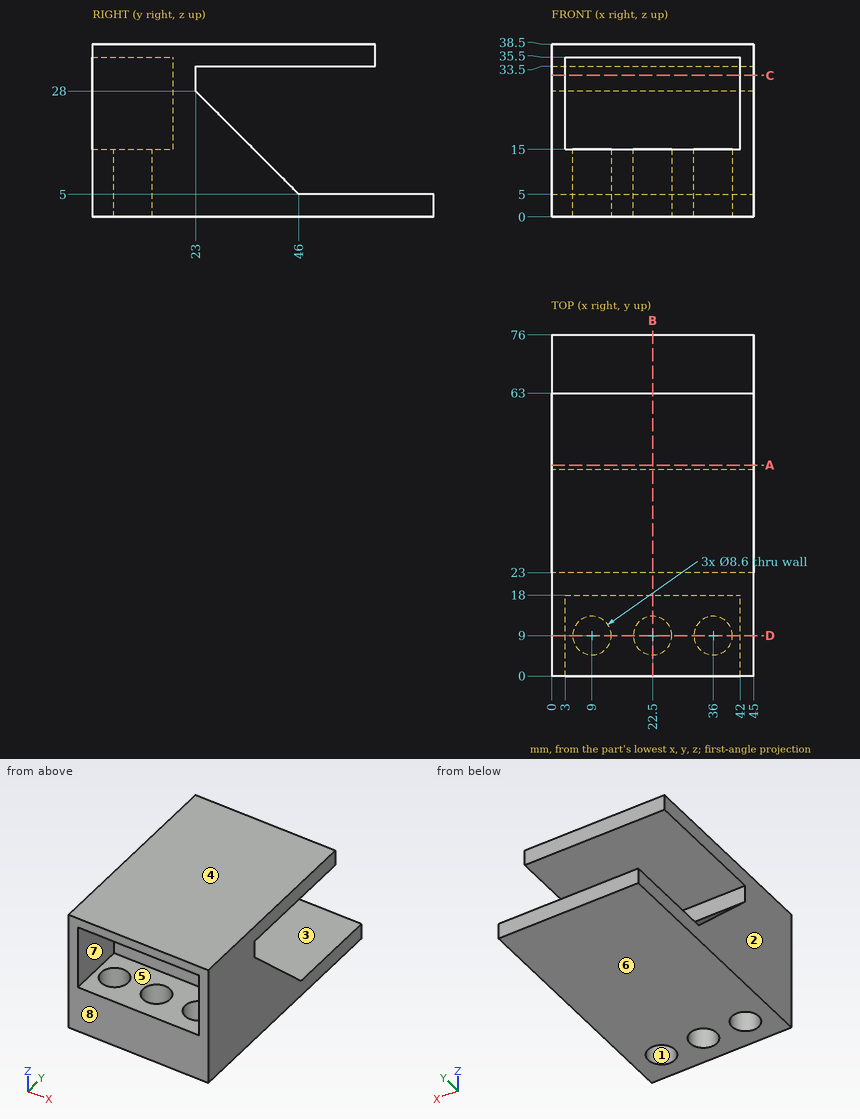
Job drawing, mm, ordinate dimensions from the low corner. One solid piece. A direction names the side the tool comes from. Give positions to 0.01 mm unless a question says otherwise; leave off trailing zeros. Order: outer loops, then holes, each group sorted by start corner. A loop starts at its lowest first (then second) coordinate and runs counter-clockwise, first axis right, second up. Notation, with made-up numbers: M -10,-0.5 L 5,-0.5 A25 cw 5,35.5 Z; hole C 17,-4 d8. An arc over 180 degrees is marked long. Return JSON: item names as keys, results as strings.
Q1. Wall check: probe 1 along Y at (x, z) = (22.5, 6); probe 2 along Z at (x, y) = (12, 61.5); probe 3 along Z at (x, y) = (38, 5). Give the ranges that are in metal, low to high. Write a range as from..to.
Answer list:
{"probe 1": "y = 0..4.7, 13.3..45", "probe 2": "z = 0..5, 33.5..38.5", "probe 3": "z = 0..15, 35.5..38.5"}
Q2. Band-saw the part on D-D (y = 9). Give the cut face in (x, z), then the cut area to 3 significant figures.
Answer list:
{"outline": "M 0,0 L 4.7,0 L 4.7,15 L 3,15 L 3,35.5 L 42,35.5 L 42,15 L 40.3,15 L 40.3,0 L 45,0 L 45,38.5 L 0,38.5 Z; M 13.3,0 L 18.2,0 L 18.2,15 L 13.3,15 Z; M 26.8,0 L 31.7,0 L 31.7,15 L 26.8,15 Z", "area": "546 mm^2"}
Q3. Band-saw the part on C-C (z = 31.5). Give the cut face in (x, y).
Answer list:
{"outline": "M 0,0 L 3,0 L 3,18 L 42,18 L 42,0 L 45,0 L 45,23 L 0,23 Z"}
Q4. Flat gauge pins, fed straight in: pin 1 (20 mm diameter, centred on x = 17, y = 13.5, fed in from -Z); pin 2 (1.5 mm diameter, centred on x = 22, z = 37, fed in from +Y); pin 3 (10 mm diameter, centred on x = 29, z = 22.5, fed in from -Y); pin 4 (8 mm diameter, centred on x = 28, z = 20, fed in from +Y). Where does each tip first touch, or does it go through?
Answer list:
{"pin 1": "stops at z = 0", "pin 2": "stops at y = 63", "pin 3": "stops at y = 18", "pin 4": "stops at y = 35"}
Q5. 3-axis set-ups, long thin cutter, end or side, ignore diameter. For the marked faces 1, 2, 3, 4 and 5: which of +Z, -Z, +X, -X, +Y, -Y reach the whole face in a straight line?
Answer list:
{"face 1": "-Z", "face 2": "+Z, -Z, -X, +Y, -Y", "face 3": "+X, -X, +Y", "face 4": "+Z, +X, -X, +Y, -Y", "face 5": "-Y"}
Q6. Band-saw the part on B-B (x = 22.5). Give the cut face in (y, z).
Answer list:
{"outline": "M 0,0 L 4.7,0 L 4.7,15 L 0,15 Z; M 0,35.5 L 18,35.5 L 18,15 L 13.3,15 L 13.3,0 L 76,0 L 76,5 L 46,5 L 23,28 L 23,33.5 L 63,33.5 L 63,38.5 L 0,38.5 Z"}
Q7. Two-plate mould, pull along Z, no slides. Class the marked faces 6, 7 and 8: pulls with the +Z half, pulls with the -Z half, needs draft (parallel to the pull), parting line crosses it, or undercut.
Answer list:
{"face 6": "pulls with the -Z half", "face 7": "undercut", "face 8": "needs draft"}
Q8. Band-saw the part on A-A (y = 47). Give the cut face in (x, z).
Answer list:
{"outline": "M 0,0 L 45,0 L 45,5 L 0,5 Z; M 0,33.5 L 45,33.5 L 45,38.5 L 0,38.5 Z"}
